from build123d import *

# Parameters (mm, degrees)
SKETCH1_W           = 8.5
SKETCH1_H           = 92.5
BOSS_EXTRUDE1_DEPTH = 10
SKETCH2_W           = 5.25
SKETCH2_H           = 90
CUT_EXTRUDE3_DEPTH  = 80
CHAMFER1_SIZE       = 2
BOSS_EXTRUDE3_DEPTH = 3.25
SKETCH9_W           = 2.05
SKETCH9_H           = 8.8
CUT_EXTRUDE4_DEPTH  = 80


with BuildPart() as part:
    # Sketch1 → Boss-Extrude1 (new body)
    with BuildSketch(Plane.XY):
        Rectangle(SKETCH1_W, SKETCH1_H)
    extrude(amount=BOSS_EXTRUDE1_DEPTH)

    # Sketch2 → Cut-Extrude3 (cut)
    with BuildSketch(Plane.XY.offset(10)):
        with Locations((-1.625, 1.25)):
            Rectangle(SKETCH2_W, SKETCH2_H)
    extrude(amount=-CUT_EXTRUDE3_DEPTH, mode=Mode.SUBTRACT)

    # Chamfer1
    chamfer1_edges = [part.edges().sort_by_distance(p)[0] for p in [
        (-4.25, -46.25, 5),
    ]]
    chamfer(chamfer1_edges, length=CHAMFER1_SIZE)

    # Sketch7 → Boss-Extrude3 (add)
    with BuildSketch(Plane.ZY.offset(-1)):
        Polygon((10, -8.75), (11, -8.75), (11, -6.95), (10.55, -6.95), (10.55, -7.75), (10, -7.75), align=None)
    boss_extrude3 = extrude(amount=-BOSS_EXTRUDE3_DEPTH)

    # Mirror2: Boss-Extrude3 across plane
    add(boss_extrude3.mirror(Plane.XY.offset(5)))

    # Sketch9 → Cut-Extrude4 (cut)
    with BuildSketch(Plane(origin=(0, 46.25, 0), x_dir=(1, 0, 0), z_dir=(0, 1, 0))):
        with Locations((2.625, -5)):
            Rectangle(SKETCH9_W, SKETCH9_H)
    extrude(amount=-CUT_EXTRUDE4_DEPTH, mode=Mode.SUBTRACT)


solid = part.part
Input: part model. Units: mm. Frame: model coordinates. A direction names the side the tool comes from. Round coordinates to 2 decimals unless told otherwise and drop trailing zeros. Order: outer loops, then holes, each group sorted by start corner. A loop starts at its lowest first (then second) coordinate and runs counter-clockwise, first axis right, second up.
1. Set-up query: faces 1 (the face through (1, 1, 5)), 2 (the face through (2, -31, 10)), 3 (the face through (1.6, 7, 5)). Return all of +Z, -Z, +X, -X, +Y, -Y with unobstructed straight access to the full face (end or side cutting, diameter ignored); none if empty.
The answers:
face 1: +Z, -Z, -X, +Y
face 2: +Z, +X, -X, -Y
face 3: +Y
2. Mould query, pull axis X, two halves, no side actions, for faces 4 (the face through (4.25, -1, 5)), 5 (the face through (2, -31, 0)), 6 (the face through (3, -33.75, 5)). Classes: released by +X, released by -X, zero draft, split by the parting line, or undercut.
The answers:
face 4: released by +X
face 5: zero draft
face 6: undercut
3. Cut plane A-A, the plane y = 1.5. Output: boundary loops of the cut face in (x, z), then the cut area to 3 significant figures.
The answers:
outline: (1, 0) - (4.25, 0) - (4.25, 10) - (1, 10) - close; hole (1.6, 0.6) - (3.65, 0.6) - (3.65, 9.4) - (1.6, 9.4) - close
area: 14.5 mm2
4. Pin query (flat end, axial travel): P1, Ø1, axis at x = 2.5, y = 10.5, coming from the +Z side; P2, Ø1, axis at y = 13, z = 9.5, coming from the -X side; P3, Ø1, axis at x = 2.5, z = 6.5, coming from the +Y side. Return the tip coordinate at first contact, or that it passes through.
The answers:
P1: stops at z = 10
P2: stops at x = 1
P3: stops at y = -33.75
5. Cut plane C-C, the plane x = -1.5. Output: boundary loops of the cut face in (y, z).
The answers:
outline: (-46.25, 0) - (-43.75, 0) - (-43.75, 10) - (-46.25, 10) - close
6. Cut plane D-D, the plane y = -35. Output: boundary loops of the cut face in (x, z).
The answers:
outline: (1, 0) - (4.25, 0) - (4.25, 10) - (1, 10) - close
7. Material intervals for line 1 (X direction, y = 12, z = 8.5); line 2 (Z direction, x = 2.75, y = -26); line 3 (Y direction, x = -0.25, z = 7), sorted ascending.
The answers:
line 1: x = 1 to 1.6, 3.65 to 4.25
line 2: z = 0 to 0.6, 9.4 to 10
line 3: y = -46.25 to -43.75
8. Cut plane B-B, the plane z = 5.75. Output: boundary loops of the cut face in (x, y), then the cut area to 3 significant figures.
The answers:
outline: (-4.25, -44.25) - (-2.25, -46.25) - (4.25, -46.25) - (4.25, 46.25) - (3.65, 46.25) - (3.65, -33.75) - (1.6, -33.75) - (1.6, 46.25) - (1, 46.25) - (1, -43.75) - (-4.25, -43.75) - close
area: 148 mm2
